Can you work these out from the drawing? Everything is in mm from the part's minimum corner. A direction names the side the tool comes from. Give positions to 0.01 mm unless a question says otherwise; leave off trailing zeros. Write each loop counter-clockwise with the first axis right and the second up, starting at its lowest first coordinate (ties: lowest second). Pieces come first, ordered by that corner, then holes. Notation, with made-up numbers: (-35, 17.25) -> (-28, 17.25) arc R23 ccw to (-28, 27.25) -> close; hole circle Ø3 at (-21.5, 66.5). An arc over 180 degrees is marked (long way). Return JSON: item names as keys, results as strings.
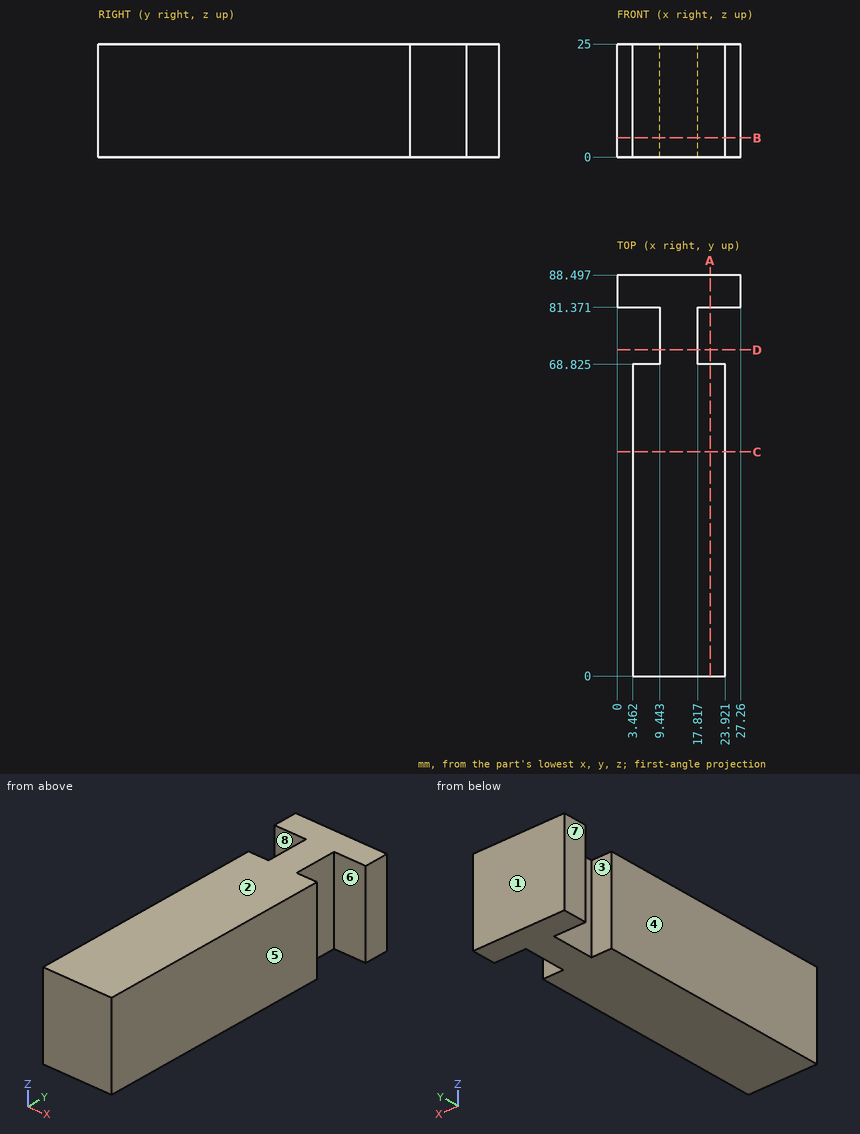
1. Suppose I cut it at B-B, the plane z = 4.25. List the corners of the cut face in (x, y) for me (1 decimal).
Taken from the geometry:
{"outline": "(0, 81.4) -> (9.4, 81.4) -> (9.4, 68.8) -> (3.5, 68.8) -> (3.5, 0) -> (23.9, 0) -> (23.9, 68.8) -> (17.8, 68.8) -> (17.8, 81.4) -> (27.3, 81.4) -> (27.3, 88.5) -> (0, 88.5) -> close"}
2. If I drill on line 1 (Y direction, x = 8.25, z = 2.5) (1 decimal); line 2 (X direction, y = 6.5, z = 15.25); line 3 (Y direction, x = 24.25, z = 10.75), over which ranges is the centre line in solid material (lowest first)? Write a range as [from, to].
Taken from the geometry:
{"line 1": "y = [0, 68.8], [81.4, 88.5]", "line 2": "x = [3.46, 23.92]", "line 3": "y = [81.37, 88.5]"}
3. Suppose I cut it at A-A, the plane x = 20.5. List the corners of the cut face in (y, z) for me (1 decimal).
Taken from the geometry:
{"outline": "(0, 0) -> (68.8, 0) -> (68.8, 25) -> (0, 25) -> close; (81.4, 0) -> (88.5, 0) -> (88.5, 25) -> (81.4, 25) -> close"}
4. Suppose I cut it at C-C, the plane y = 49.5. List the corners of the cut face in (x, z) for me.
Taken from the geometry:
{"outline": "(3.46, 0) -> (23.92, 0) -> (23.92, 25) -> (3.46, 25) -> close"}
5. Which directions (+Z, -Z, +X, -X, +Y, -Y) give clear straight access to the entire face, cutting with the end or side of a thin tool? Please do the marked faces 4, 5, 6, 7 and 8.
Taken from the geometry:
{"face 4": "+Z, -Z, -X, -Y", "face 5": "+Z, -Z, +X, -Y", "face 6": "+Z, -Z, +X", "face 7": "+Z, -Z, -X, +Y, -Y", "face 8": "+Z, -Z, -X"}
6. If we mould it in two halves opening along Y, with no side actions, what happens to the marked faces 1, 2 and 3? For each: released by +Y, released by -Y, zero draft, split by the parting line, or undercut.
Taken from the geometry:
{"face 1": "released by +Y", "face 2": "zero draft", "face 3": "undercut"}
7. For pin 1 Ø1 at (y, z) = (57.5, 10) entering from -X; pin 2 Ø8 at (y, z) = (9.5, 19) entering from +X; pin 3 Ø4 at (y, z) = (72.5, 10.5) entering from -X; pin 4 Ø10.5 at (x, z) = (22, 10) entering from -Y, each with a flat end and sliding along its axis, tell me the tip position at first contact or that it passes through.
Taken from the geometry:
{"pin 1": "stops at x = 3.46", "pin 2": "stops at x = 23.92", "pin 3": "stops at x = 9.44", "pin 4": "stops at y = 0"}
8. Suppose I cut it at D-D, the plane y = 72. List the corners of the cut face in (x, z) for me, and give its area (3 significant figures).
Taken from the geometry:
{"outline": "(9.44, 0) -> (17.82, 0) -> (17.82, 25) -> (9.44, 25) -> close", "area": "209 mm²"}
